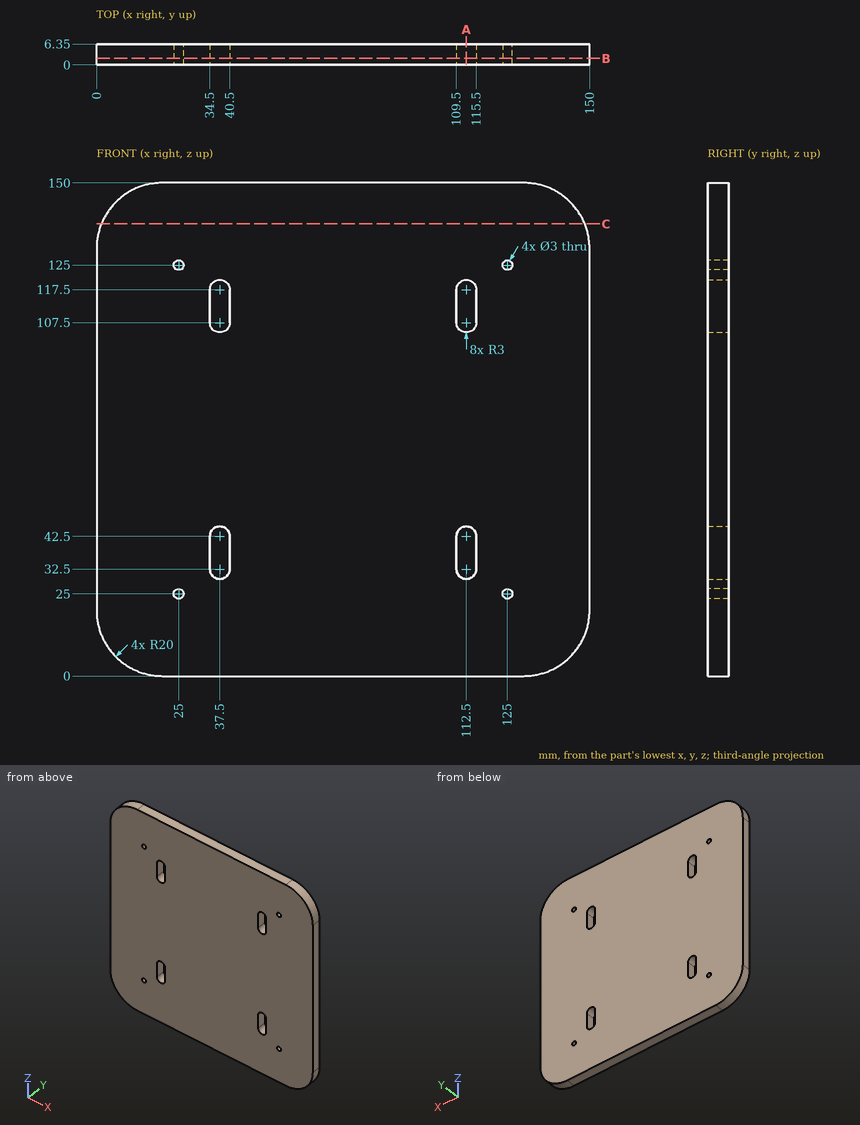
Geometry: see drawing. Coordinates: mm, zero at the bounding-box minimum. Round coordinates to 2 decimals unless told otherwise and drop trailing zeros. Write each loop counter-clockwise with the first axis right and the second up, starting at its lowest first coordinate (ties: lowest second). Pieces come first, ordered by that corner, then holes. Notation, with made-up numbers: (-21.75, -11) -> (33.25, -11) arc R27 cw to (33.25, 10) -> close; hole circle Ø6 at (-15.5, 49). An arc over 180 degrees is marked (long way). Answer as CSV lines item,"result".
1. Contact query for a flat-ended pin moving along its axis: P1, Ø1.8, axis at x = 25, z = 25, coming from the -Y side. Output: stop coordinate, or through.
Geometry says:
P1,"passes through"
2. Ray query, L1, parallel to X at y = 1.5, z = 125; L2, parallel to X at y = 4.75, z = 116.5. Return the intervals inside material, ascending. Write a range as [from, to].
Geometry says:
L1,"x = [0, 23.5], [26.5, 123.5], [126.5, 150]"
L2,"x = [0, 34.5], [40.5, 109.5], [115.5, 150]"
3. Section C-C (z = 137.5). Return the cut outline in (x, y).
Geometry says:
outline,"(1.46, 0) -> (148.54, 0) -> (148.54, 6.35) -> (1.46, 6.35) -> close"
4. Section A-A (x = 112.5). Return the cut outline in (y, z), plus the area to 3 significant figures.
Geometry says:
outline,"(0, 0) -> (6.35, 0) -> (6.35, 29.5) -> (0, 29.5) -> close; (0, 45.5) -> (6.35, 45.5) -> (6.35, 104.5) -> (0, 104.5) -> close; (0, 120.5) -> (6.35, 120.5) -> (6.35, 150) -> (0, 150) -> close"
area,"749 mm^2"
5. Section B-B (y = 2). Give the number of separate pieces and of enclosed holes in the cut face, plus the area to 3 significant figures.
Geometry says:
separate pieces,"1"
enclosed holes,"8"
area,"21,800 mm^2"
